from build123d import *

# Parameters (mm, degrees)
SKETCH1_W           = 18
SKETCH1_H           = 220
BOSS_EXTRUDE1_DEPTH = 9.8
SKETCH3_R           = 1.75
CUT_EXTRUDE1_DEPTH  = 35
SKETCH4_R           = 2.75
CUT_EXTRUDE2_DEPTH  = 4


with BuildPart() as part:
    # Sketch1 → Boss-Extrude1 (new body)
    with BuildSketch(Plane(origin=(0, 0, 0), x_dir=(1, 0, 0), z_dir=(0, 1, 0))):
        Rectangle(SKETCH1_W, SKETCH1_H)
    extrude(amount=BOSS_EXTRUDE1_DEPTH)

    # Sketch3 → Cut-Extrude1 (cut)
    with BuildSketch(Plane.ZY.offset(9)):
        with Locations((-104.5, 4.9)):
            Circle(SKETCH3_R)
        with Locations((104.5, 4.9)):
            Circle(SKETCH3_R)
    extrude(amount=-CUT_EXTRUDE1_DEPTH, mode=Mode.SUBTRACT)

    # Sketch4 → Cut-Extrude2 (cut)
    with BuildSketch(Plane.ZY.offset(9)):
        with Locations((-104.5, 4.9)):
            Circle(SKETCH4_R)
        with Locations((104.5, 4.9)):
            Circle(SKETCH4_R)
    extrude(amount=-CUT_EXTRUDE2_DEPTH, mode=Mode.SUBTRACT)


solid = part.part
Design review of the part built by this model. Coordinates are the model's own, in mm. A direction names the side the tool comes from. Round coordinates to 2 decimals unless told otherwise and drop trailing zeros. Write each loop counter-clockwise with the first axis right and the second up, starting at its lowest first coordinate (ties: lowest second). Pieces come first, ordered by that corner, then holes. Notation, with made-up numbers: (14, 78) -> (61, 78) arc R7 ccw to (61, 86) -> close; hole circle Ø9 at (-17, 47.25). An arc over 180 degrees is marked (long way). One line per item, written item: value. Start each with the question number.
Q1. Tool access review of faces 4 (the face through (0, 0, -2)), 5 (the face through (-7.028, 5.021, 101.753)): name each direction out of +Z, -Z, +X, -X, +Y, -Y from which nothing blocks a thin tool from reaching the whole face with its end or side.
Q2. Insertion check: P1, Ø3, axis at y = 4.9, z = 104.5, coming from the +X side; P2, Ø3, axis at y = 5, z = 104, coming from the -X side. Each pin has a flat end and moves straight along its axis. Give the tip position at first contact, or say it passes through.
Q3. Add section A-A (y = 4.9). Give the boundary of the cut face in (x, z).
Q4. The part is to be moulded in two halves that separate along Z. For faces 1 (the face through (9, 5, 2)), 2 (the face through (0, 5, -110)), 3 (the face through (-5, 3, 104)), say which applies: pulls with the +Z half, pulls with the -Z half, needs draft (parallel to the pull), parting line crosses it, or undercut.
Q5. To check wall thickness, follow probe 1 along Z at (x, y) = (4.5, 5); probe 2 along Y at (x, z) = (-7.95, -104.5); probe 3 along Z at (x, y) = (-7, 2.5). State the ranges of each line that lie inside material, in increasing order.
Response:
1. face 4: +Z, -Z, +X, -X, -Y
1. face 5: -X
2. P1: passes through
2. P2: stops at x = -5
3. outline: (-9, -110) -> (9, -110) -> (9, -106.25) -> (-5, -106.25) -> (-5, -107.25) -> (-9, -107.25) -> close; (-9, -101.75) -> (-5, -101.75) -> (-5, -102.75) -> (9, -102.75) -> (9, 102.75) -> (-5, 102.75) -> (-5, 101.75) -> (-9, 101.75) -> close; (-9, 107.25) -> (-5, 107.25) -> (-5, 106.25) -> (9, 106.25) -> (9, 110) -> (-9, 110) -> close
4. face 1: needs draft
4. face 2: pulls with the -Z half
4. face 3: undercut
5. probe 1: z = -110 to -106.25, -102.75 to 102.75, 106.25 to 110
5. probe 2: y = 0 to 2.15, 7.65 to 9.8
5. probe 3: z = -110 to -105.84, -103.16 to 103.16, 105.84 to 110
